Verification items for the finished model (mm, model axes). Round coordinates to 2 decimals unless told otherwise and drop trailing zeros. Order: outer loops, then holes, each group sorted by start corner. A loop starts at its lowest first (then second) coordinate and runs counter-clockwise, first axis right, second up. Notation, with made-up numbers: M 21.5,71 L 48.5,71 A13 ccw 48.5,92 Z; hole C 86,76.25 d10. An arc over 180 degrees is marked long. Answer as a JSON object with one key per item and string values. Group by question number.
```python
from build123d import *

# Parameters (mm, degrees)
SKETCH1_R              = 14.2875
BOSS_EXTRUDE1_DEPTH    = 1.5875
F_10_CLEARANCE_HOLE1_D = 4.9784
FILLET1_R              = 12.7


with BuildPart() as part:
    # Sketch1 → Boss-Extrude1 (new body)
    with BuildSketch(Plane.XY):
        with BuildLine():
            Line((0, 22.225), (22.225, 22.225))
            Line((22.225, 22.225), (45.6057, 28.575))
            Line((45.6057, 28.575), (134.5057, 28.575))
            Line((134.5057, 28.575), (157.8864, 22.225))
            Line((157.8864, 22.225), (180.1114, 22.225))
            ThreePointArc((180.1114, 22.225), (202.3364, 0), (180.1114, -22.225))
            Line((180.1114, -22.225), (157.8864, -22.225))
            Line((157.8864, -22.225), (134.5057, -28.575))
            Line((134.5057, -28.575), (45.6057, -28.575))
            Line((45.6057, -28.575), (22.225, -22.225))
            Line((22.225, -22.225), (0, -22.225))
            ThreePointArc((0, -22.225), (-22.225, 0), (0, 22.225))
        make_face()
        Circle(SKETCH1_R, mode=Mode.SUBTRACT)
        with Locations((180.1114, 0)):
            Circle(SKETCH1_R, mode=Mode.SUBTRACT)
    extrude(amount=BOSS_EXTRUDE1_DEPTH)

    # #10 Clearance Hole1 (through all)
    with Locations(Plane.XY.offset(1.5875)):
        with Locations((64.6557, -22.225), (27.7114, 0), (64.6557, 22.225), (90.0557, 22.225), (53.1114, 0), (78.5114, 0), (101.6, 0), (127, 0), (115.4557, 22.225), (152.4, 0), (115.4557, -22.225), (90.0557, -22.225)):
            Hole(F_10_CLEARANCE_HOLE1_D / 2)

    # Fillet1
    fillet1_edges = [part.edges().sort_by_distance(p)[0] for p in [
        (22.225, 22.225, 0.79375),
        (45.6057, 28.575, 0.79375),
        (134.5057, 28.575, 0.79375),
        (157.8864, 22.225, 0.79375),
        (157.8864, -22.225, 0.79375),
        (134.5057, -28.575, 0.79375),
        (45.6057, -28.575, 0.79375),
        (22.225, -22.225, 0.79375),
    ]]
    fillet(fillet1_edges, radius=FILLET1_R)


solid = part.part
```
Q1. Gauge pin test, flat end, axial feed: pin 1 Ø0.8 at (x, z) = (10.5, 0.5) entering from -Y (3 decimals). Record the tip position at first contact, or that the pin passes through.
Q2. Cross-section at B-B, the plane z = 0.4. Give the number of separate pieces and of enclosed holes in the cut face, then the cut area to 3 significant figures.
Q3. Thickness scan on line 1 (Y direction, x = 127, z = 0.6) (3 decimals); line 2 (X direction, y = -3, z = 0.95); line 3 (Y direction, x = -1, z = 0.45). Record the ranges inside material, lowest first. Write a range as from..to.
Q4. Cross-section at D-D, the plane x = 152.4. Record the cut outline in (y, z), then the cut area to 3 significant figures.
Q5. Release check for a two-part mould opening along Y. For faces 1 (the face through (146.055, 25.438, 0.783)), 2 (the face through (92, 0, 1.588)), 3 (the face through (113.08, -21.48, 0.78)) record: released by +Y, released by -Y, zero draft, split by the parting line, or undercut.
Q6. Cross-section at A-A, the plane x = 101.6. Record the cut outline in (y, z) (1 decimal).
Conclusion:
{
 "1": {"pin 1": "y = -22.225"},
 "2": {"separate pieces": "1", "enclosed holes": "14", "area": "9,470 mm2"},
 "3": {"line 1": "-28.575..-2.489, 2.489..28.575", "line 2": "-22.02..-13.97, 13.97..166.14, 194.08..202.13", "line 3": "-22.2..-14.25, 14.25..22.2"},
 "4": {"outline": "M -23.72,0 L -2.49,0 L -2.49,1.59 L -23.72,1.59 Z; M 2.49,0 L 23.72,0 L 23.72,1.59 L 2.49,1.59 Z", "area": "67.4 mm2"},
 "5": {"face 1": "released by +Y", "face 2": "zero draft", "face 3": "undercut"},
 "6": {"outline": "M -28.6,0 L -2.5,0 L -2.5,1.6 L -28.6,1.6 Z; M 2.5,0 L 28.6,0 L 28.6,1.6 L 2.5,1.6 Z"}
}
